Can you work these out from the model? Positions are in its coordinate system, mm. Face numbers are marked on the shaded views. A direction names the side the tool comes from. Coordinates: 2 decimals unless noted, no trailing zeros. Order: outer loops, then holes, each group sorted by start corner. A loop starts at its lowest first (then second) coordinate and runs counter-clockwise, first axis right, second up. Notation, with made-up numbers: (59, 48) -> (88, 48) arc R4 cw to (88, 54) -> close; hole circle Ø6 at (-1.75, 68.25). An arc over 180 degrees is marked (long way). Answer as CSV lines item,"result".
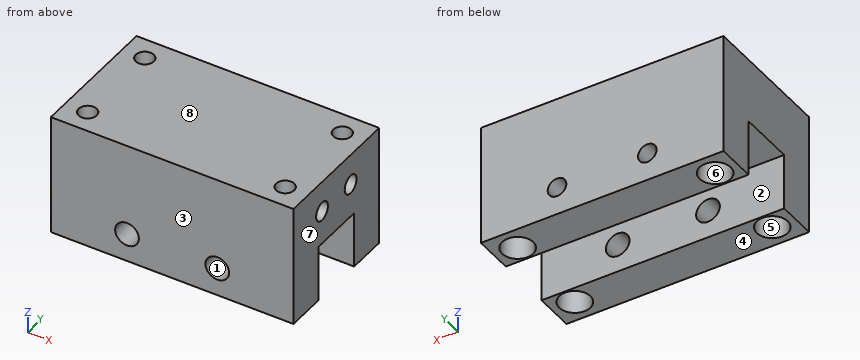
from build123d import *

# Parameters (mm, degrees)
SKETCH_1_W             = 43
SKETCH_1_H             = 24
SKETCH_1_R             = 1.6
EXTRUDE_1_DEPTH        = 11.5
SKETCH_3_W             = 43
SKETCH_3_H             = 7
SKETCH_3_R             = 2.75
EXTRUDE_2_DEPTH        = 10
CUT_EXTRUDE_START      = -15
SKETCH_4_R             = 2.1
CUT_EXTRUDE_1_DEPTH    = 10
HOLE_WIZARD_M4_1_D     = 3.3
HOLE_WIZARD_M4_1_DEPTH = 10.1
HOLE_WIZARD_M4_1_TIP   = 0.991420021
HOLE_WIZARD_M4_2_D     = 3.3
HOLE_WIZARD_M4_2_DEPTH = 10.1
HOLE_WIZARD_M4_2_TIP   = 0.991420021


with BuildPart() as part:
    # 草图1 → 凸台-拉伸1 (new body)
    with BuildSketch(Plane.XY):
        Rectangle(SKETCH_1_W, SKETCH_1_H)
        with Locations((-17.5, 8)):
            Circle(SKETCH_1_R, mode=Mode.SUBTRACT)
        with Locations((-17.5, -8)):
            Circle(SKETCH_1_R, mode=Mode.SUBTRACT)
        with Locations((17.5, -8)):
            Circle(SKETCH_1_R, mode=Mode.SUBTRACT)
        with Locations((17.5, 8)):
            Circle(SKETCH_1_R, mode=Mode.SUBTRACT)
    extrude(amount=EXTRUDE_1_DEPTH)

    # 草图3 → 凸台-拉伸2 (add)
    # profile 1 of 2: a face of its own
    with BuildSketch(Plane(origin=(0, 0, 0), x_dir=(-1, 0, 0), z_dir=(0, 0, -1))):
        with Locations((0, -8.5)):
            Rectangle(SKETCH_3_W, SKETCH_3_H)
        with Locations((-17.5, -8)):
            Circle(SKETCH_3_R, mode=Mode.SUBTRACT)
        with Locations((17.5, -8)):
            Circle(SKETCH_3_R, mode=Mode.SUBTRACT)
    # profile 2 of 2: a face of its own
    with BuildSketch(Plane(origin=(0, 0, 0), x_dir=(-1, 0, 0), z_dir=(0, 0, -1))):
        with Locations((0, 8.5)):
            Rectangle(SKETCH_3_W, SKETCH_3_H)
        with Locations((17.5, 8)):
            Circle(SKETCH_3_R, mode=Mode.SUBTRACT)
        with Locations((-17.5, 8)):
            Circle(SKETCH_3_R, mode=Mode.SUBTRACT)
    extrude(amount=EXTRUDE_2_DEPTH)

    # 草图4 → 切除-拉伸1 (cut)
    with BuildSketch(Plane(origin=(0, 12, 0), x_dir=(1, 0, 0), z_dir=(0, 1, 0)).offset(CUT_EXTRUDE_START)):
        with Locations(Location((8, 5, 0), (0, 0, 180))):
            Circle(SKETCH_4_R)
        with Locations(Location((-8, 5, 0), (0, 0, 180))):
            Circle(SKETCH_4_R)
    extrude(amount=-CUT_EXTRUDE_1_DEPTH, mode=Mode.SUBTRACT)

    # M4 螺纹孔1
    with Locations(Plane(origin=(0, 12, 0), x_dir=(1, 0, 0), z_dir=(0, 1, 0))):
        with Locations((-8, 5), (8, 5)):
            Hole(HOLE_WIZARD_M4_1_D / 2, depth=HOLE_WIZARD_M4_1_DEPTH)
            with Locations((0, 0, -(HOLE_WIZARD_M4_1_DEPTH + HOLE_WIZARD_M4_1_TIP / 2))):  # 118° drill point
                Cone(0, HOLE_WIZARD_M4_1_D / 2, HOLE_WIZARD_M4_1_TIP, mode=Mode.SUBTRACT)

    # M4 螺纹孔2
    with Locations(Plane(origin=(21.5, 4, 6), x_dir=(0, 1, 0), z_dir=(1, 0, 0))):
        with Locations((0, 0), (-8, 0)):
            Hole(HOLE_WIZARD_M4_2_D / 2, depth=HOLE_WIZARD_M4_2_DEPTH)
            with Locations((0, 0, -(HOLE_WIZARD_M4_2_DEPTH + HOLE_WIZARD_M4_2_TIP / 2))):  # 118° drill point
                Cone(0, HOLE_WIZARD_M4_2_D / 2, HOLE_WIZARD_M4_2_TIP, mode=Mode.SUBTRACT)


solid = part.part
Q1. Which directions (+Z, -Z, +X, -X, +Y, -Y) give clear straight access to the entire face, cutting with the end or side of a thin tool? Please do the marked faces 1, 2, 3, 4 and 5.
Solution:
face 1,"-Y"
face 2,"-Z, +X, -X"
face 3,"+Z, -Z, +X, -X, -Y"
face 4,"-Z, +X, -X, +Y, -Y"
face 5,"-Z"
Q2. We'd pull the mould along X, two halves only. Please class the marked faces 6, 7 and 8: pulls with the +X half, pulls with the -X half, needs draft (parallel to the pull), parting line crosses it, or undercut.
Solution:
face 6,"undercut"
face 7,"pulls with the +X half"
face 8,"needs draft"
Q3. Imagine slicing it at D-D (z = -5). Give the number of separate pieces and of enclosed holes in the cut face, and give its area (3 significant figures).
Solution:
separate pieces,"6"
enclosed holes,"4"
area,"402 mm2"
Q4. If I drill on line 1 (Y direction, x = -17.5, z = -4.5); line 2 (Y direction, x = 1, z = -8.25); line 3 (X direction, y = 9, z = -7), over which ranges is the centre line in solid material (lowest first)?
Solution:
line 1,"-12 to -10.75, -5.25 to -5, 5 to 5.25, 10.75 to 12"
line 2,"-12 to -5, 5 to 12"
line 3,"-21.5 to -20.06, -14.94 to 14.94, 20.06 to 21.5"
Q5. For P1, Ø2.5, axis at y = -4, z = 6, coming from the +X side; P2, Ø3, axis at y = 4, z = 6, coming from the +X side; P3, Ø3.5, axis at x = 17.5, y = 8, coming from the -Z side; P4, Ø3, axis at x = -17.5, y = 8, coming from the +Z side, each with a flat end and sliding along its axis, tell me the tip position at first contact or that it passes through.
Solution:
P1,"x = 11.16"
P2,"x = 11.31"
P3,"z = 0"
P4,"through"
Q6. Imagine slicing it at B-B (z = -8.5). List the corners of the cut face in (x, y) for me.
Solution:
outline,"(-21.5, -12) -> (21.5, -12) -> (21.5, -5) -> (-21.5, -5) -> close; (-21.5, 5) -> (21.5, 5) -> (21.5, 12) -> (-21.5, 12) -> close; hole circle Ø5.5 at (-17.5, -8); hole circle Ø5.5 at (-17.5, 8); hole circle Ø5.5 at (17.5, -8); hole circle Ø5.5 at (17.5, 8)"
Q7. Imagine slicing it at A-A (y = 8). List the corners of the cut face in (x, z) for me.
Solution:
outline,"(-21.5, -10) -> (-20.25, -10) -> (-20.25, 0) -> (-19.1, 0) -> (-19.1, 11.5) -> (-21.5, 11.5) -> close; (-15.9, 0) -> (-14.75, 0) -> (-14.75, -10) -> (14.75, -10) -> (14.75, 0) -> (15.9, 0) -> (15.9, 11.5) -> (-15.9, 11.5) -> close; (19.1, 0) -> (20.25, 0) -> (20.25, -10) -> (21.5, -10) -> (21.5, 11.5) -> (19.1, 11.5) -> close; hole circle Ø3.3 at (-8, -5); hole circle Ø3.3 at (8, -5)"
Q8. Imagine slicing it at C-C (x = 12.5). List the corners of the cut face in (y, z) for me, and give its area (3 significant figures).
Solution:
outline,"(-12, -10) -> (-5, -10) -> (-5, 0) -> (5, 0) -> (5, -10) -> (12, -10) -> (12, 11.5) -> (-12, 11.5) -> close; hole circle Ø3.3 at (-4, 6); hole circle Ø3.3 at (4, 6)"
area,"399 mm2"
